```python
from build123d import *

# Parameters (mm, degrees)
ESBO_O2_W                = 18
ESBO_O2_H                = 80
RESSALTO_EXTRUS_O1_DEPTH = 80
CASCA1_T                 = -3
ESBO_O4_R                = 1.6
ESBO_O4_R_2              = 6
ESBO_O4_R_3              = 3.5
ESBO_O4_R_4              = 6.25
ESBO_O4_W                = 100
ESBO_O4_H                = 40
CORTE_EXTRUS_O1_DEPTH    = 3
ESBO_O5_R                = 1.6
RESSALTO_EXTRUS_O2_DEPTH = 160
ESBO_O6_W                = 45
ESBO_O6_H                = 12
CORTE_EXTRUS_O2_DEPTH    = 19
ESBO_O7_W                = 12
ESBO_O7_H                = 40
CORTE_EXTRUS_O3_DEPTH    = 10
CHANFRO1_SIZE            = 5
CHANFRO1_SIZE2           = 2.886751346


with BuildPart() as part:
    # Esboço2 → Ressalto-extrusão1 (new body, symmetric)
    with BuildSketch(Plane(origin=(0, 0, 0), x_dir=(0, 0, -1), z_dir=(1, 0, 0))):
        with Locations((9, 40)):
            Rectangle(ESBO_O2_W, ESBO_O2_H)
    extrude(amount=RESSALTO_EXTRUS_O1_DEPTH, both=True)

    # Casca1
    casca1_openings = [part.faces().sort_by_distance(p)[0] for p in [
        (0, 40, 0),
    ]]
    offset(amount=CASCA1_T, openings=casca1_openings, kind=Kind.INTERSECTION)

    # Esboço4 → Corte-extrusão1 (cut)
    with BuildSketch(Plane(origin=(0, 0, -18), x_dir=(1, 0, 0), z_dir=(0, 0, -1))):
        with Locations((-72, -24)):
            Circle(ESBO_O4_R)
        with Locations((-72, -73)):
            Circle(ESBO_O4_R)
        with Locations((72, -73)):
            Circle(ESBO_O4_R)
        with Locations((72, -24)):
            Circle(ESBO_O4_R)
        with Locations((-62, -47)):
            Circle(ESBO_O4_R_2)
        with Locations((-61.5, -29)):
            Circle(ESBO_O4_R_3)
        with Locations((-62, -66)):
            Circle(ESBO_O4_R_4)
        with Locations((11.5, -44)):
            Rectangle(ESBO_O4_W, ESBO_O4_H)
    extrude(amount=-CORTE_EXTRUS_O1_DEPTH, mode=Mode.SUBTRACT)

    # Esboço5 → Ressalto-extrusão2 (add, through all)
    with BuildSketch(Plane(origin=(80, 0, 0), x_dir=(0, 0, -1), z_dir=(1, 0, 0))):
        with BuildLine():
            Line((14.538461538, 88.307692308), (18, 80))
            Line((18, 80), (0, 80))
            Line((0, 80), (3.461538462, 88.307692308))
            ThreePointArc((3.461538462, 88.307692308), (9, 92), (14.538461538, 88.307692308))
        make_face()
        with Locations((9, 86)):
            Circle(ESBO_O5_R, mode=Mode.SUBTRACT)
    extrude(amount=-RESSALTO_EXTRUS_O2_DEPTH)

    # Esboço6 → Corte-extrusão2 (cut, through all)
    with BuildSketch(Plane(origin=(0, 0, -18), x_dir=(-1, 0, 0), z_dir=(0, 0, -1))):
        with Locations((-57.5, 86)):
            Rectangle(ESBO_O6_W, ESBO_O6_H)
        with Locations((57.5, 86)):
            Rectangle(ESBO_O6_W, ESBO_O6_H)
    extrude(amount=-CORTE_EXTRUS_O2_DEPTH, mode=Mode.SUBTRACT)

    # Esboço7 → Corte-extrusão3 (cut)
    with BuildSketch(Plane(origin=(80, 0, 0), x_dir=(0, 0, -1), z_dir=(1, 0, 0))):
        with Locations((6, 40)):
            Rectangle(ESBO_O7_W, ESBO_O7_H)
    extrude(amount=-CORTE_EXTRUS_O3_DEPTH, mode=Mode.SUBTRACT)

    # Chanfro1
    chanfro1_edges = [part.edges().sort_by_distance(p)[0] for p in [
        (80, 40, -12),
    ]]
    chanfro1_side = [part.faces().sort_by_distance(p)[0] for p in [
        (80, 79.18, -9),
    ]]
    chamfer(chanfro1_edges, length=CHANFRO1_SIZE, length2=CHANFRO1_SIZE2, reference=chanfro1_side[0])


solid = part.part
```
Geometry: final body of the model. Coordinates: model frame, mm. A direction names the side the tool comes from. Coordinates: 2 decimals unless noted, no trailing zeros. Order: outer loops, then holes, each group sorted by start corner. A loop starts at its lowest first (then second) coordinate and runs counter-clockwise, first axis right, second up. Notation, with made-up numbers: (-18.75, -38) - (36.25, -38) arc R14 cw to (36.25, -26) - close; hole circle Ø9 at (-19, 14). An arc over 180 degrees is marked (long way). Write each question's results on one line, items separated by ' | '.
(1) Line query: line 1 (Y direction, x = 72, z = -16.85); line 2 (Y direction, x = -62, z = -16.5); line 3 (X direction, y = 73, z = -16.15). Output: solid intervals per line, ascending. Write a range as [from, to].
Values found:
line 1: y = [0, 22.4], [25.6, 71.4], [74.6, 80] | line 2: y = [0, 25.54], [32.46, 41], [53, 59.75], [72.25, 80] | line 3: x = [-80, -73.6], [-70.4, 70.4], [73.6, 80]
(2) Section query C-C, the plane x = -21.5. Return the cut outline in (y, z), plus the area to 3 significant figures.
Values found:
outline: (0, -18) - (24, -18) - (24, -15) - (3, -15) - (3, 0) - (0, 0) - close; (64, -18) - (80, -18) - (88.31, -14.54) arc R6 ccw to (88.31, -3.46) - (80, 0) - (77, 0) - (77, -15) - (64, -15) - close; hole circle Ø3.2 at (86, -9) | area: 352 mm²
(3) First-contact query: pin 1 Ø3.5 at (y, z) = (83.5, -13) entering from -X; pin 2 Ø2.5 at (x, y) = (72, 24) entering from +Z; pin 3 Ø5.5 at (x, z) = (-58.5, -11) entering from +Y; pin 4 Ø3 at (x, z) = (-0.5, -2.5) entering from +Y. Flat tips, straight axial feed; report the tip coordinate or a pass-through.
Values found:
pin 1: stops at x = -35 | pin 2: passes through | pin 3: stops at y = 80 | pin 4: stops at y = 89.32
(4) Section query A-A, the plane x = -72. Return the cut outline in (y, z), plus the area to 3 significant figures.
Values found:
outline: (0, -18) - (22.4, -18) - (22.4, -15) - (3, -15) - (3, 0) - (0, 0) - close; (25.6, -18) - (71.4, -18) - (71.4, -15) - (25.6, -15) - close; (74.6, -18) - (80, -18) - (80, 0) - (77, 0) - (77, -15) - (74.6, -15) - close | area: 311 mm²
(5) Section query B-B, the plane y = 47. Return the cut outline in (x, z), plus the area to 3 significant figures.
Values found:
outline: (-80, -18) - (-68, -18) - (-68, -15) - (-77, -15) - (-77, 0) - (-80, 0) - close; (-56, -18) - (-38.5, -18) - (-38.5, -15) - (-56, -15) - close; (61.5, -18) - (80, -18) - (80, -17) - (77.11, -12) - (77, -12) - (77, -15) - (61.5, -15) - close | area: 191 mm²
(6) Section query D-D, the plane y = 66. Return the cut outline in (x, z).
Values found:
outline: (-80, -18) - (-68.25, -18) - (-68.25, -15) - (-77, -15) - (-77, 0) - (-80, 0) - close; (-55.75, -18) - (80, -18) - (80, 0) - (77, 0) - (77, -15) - (-55.75, -15) - close
(7) Mould query, pull axis Y, two halves, no side actions, for faces 1 (the face through (35, 83, -9)), 2 (the face through (58, 80, -9)), 3 (the face through (79, 20, -6)). Classes: +Y half, -Y half, draft (parallel to the pull), parting line (faces both ways), or undercut.
Values found:
face 1: draft | face 2: +Y half | face 3: undercut
(8) Set-up query: faces 4 (the face through (0.49, 84.1, -1.71)), 5 (the face through (-35, 83, -9)), 6 (the face through (11, 64, -17)), 7 (the face through (1, 3, -7)). Return all of +Z, -Z, +X, -X, +Y, -Y with unobstructed straight access to the full face (end or side cutting, diameter ignored); none if empty.
Values found:
face 4: +Z, +X, -X, +Y | face 5: +Z, -Z, -X, +Y | face 6: +Z, -Z | face 7: +Z
